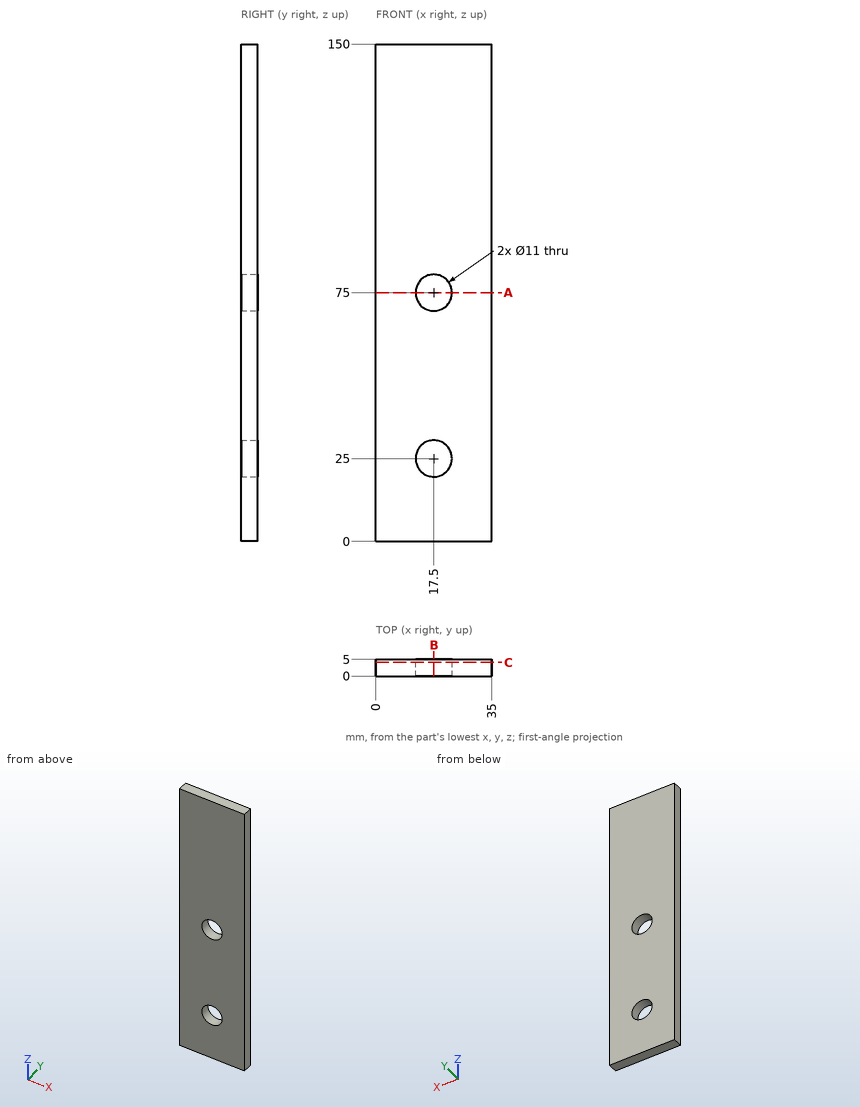
Source: three-view drawing plus pictorial views. Frame: mm from the lowest corner of the part. Give positions to 0.01 mm unless a question says otherwise; leave off trailing zeros. Loops run counter-clockwise (first coordinate to the right, second up) from the corner with the lowest first, then second, coordinate; pieces in that order, holes last. Notation, with made-up numbers: M 1,28.25 L 48,28.25 A20 ccw 48,39.25 Z; hole C 40.5,65 d5. An arc over 180 degrees is marked long. Use CSV: the item, a comma, the result in double quotes.
(1) Material intervals for L1, parallel to Z at x = 17.5, y = 2.2; L2, parallel to Z at x = 21.5, y = 0.85; L3, parallel to X at y = 4.5, z = 78, sorted ascending. Write a range as [from, to].
Outcome:
L1,"z = [0, 19.5], [30.5, 69.5], [80.5, 150]"
L2,"z = [0, 21.23], [28.77, 71.23], [78.77, 150]"
L3,"x = [0, 12.89], [22.11, 35]"
(2) Section C-C, the plane y = 4.1. Return loops of the section in (x, z).
Outcome:
outline,"M 0,0 L 35,0 L 35,150 L 0,150 Z; hole C 17.5,25 d11; hole C 17.5,75 d11"
(3) Section B-B, the plane x = 17.5. Return loops of the section in (y, z).
Outcome:
outline,"M 0,0 L 5,0 L 5,19.5 L 0,19.5 Z; M 0,30.5 L 5,30.5 L 5,69.5 L 0,69.5 Z; M 0,80.5 L 5,80.5 L 5,150 L 0,150 Z"
(4) Pin query (flat end, axial travel): P1, Ø6.5, axis at x = 17.5, z = 75, coming from the +Y side. Return the tip coordinate at first contact, or that it passes through.
Outcome:
P1,"passes through"
(5) Section A-A, the plane z = 75. Return loops of the section in (x, y).
Outcome:
outline,"M 0,0 L 12,0 L 12,5 L 0,5 Z; M 23,0 L 35,0 L 35,5 L 23,5 Z"
